Source: CAD feature listing. Evaluate the final solid. Frame: model axes, mm. A direction names the side the tool comes from. Round coordinates to 2 decimals unless told otherwise and drop trailing zeros. Loops run counter-clockwise (first coordinate to the right, second up) from the corner with the lowest first, then second, coordinate; pieces in that order, holes last. Notation, with made-up numbers: (60.5, 23.25) - (118.5, 23.25) arc R37 ccw to (118.5, 60.25) - close; hole circle Ø4 at (6.25, -29.75). An arc over 180 degrees is marked (long way). One line per question, with ' | ' between items. Start each with the question number.
1. Cut plane A-A (x = 0). Return loops of the section in (y, z).
2. Access query for faces 4 (the flat face through (0, 4.636, 41)), 5 (the cylindrical face through (0.255, -6.345, 41.497)), 6 (the cylindrical face through (3.094, -2.372, 15.653)). Directions: +Z, -Z, +X, -X, +Y, -Y. A direction counts if a zero-diameter tool reaches every point of the face in a straight line with its end or side. Return the directions, or none.
3. Ray query, line 1 (Y direction, x = 0, z = 21); line 2 (Z direction, x = -0.25, y = 7.25); line 3 (Z direction, x = 1, y = -1.5). Return the intervals inside material, ascending.
4. Cut plane B-B (y = 0). Return loops of the section in (x, z).
5. Pin query (flat end, axial travel): pin 1 (2.5 mm diameter, centred on x = -0.5, z = 37.5, fed in from +Y); pin 2 (3 mm diameter, centred on y = -1, z = 28, fed in from -X); pin 3 (0.7 mm diameter, centred on y = 5.5, z = 35.5, fed in from +X). Return the tip coordinate at first contact, or that it passes through.
6. Mould query, pull axis Y, two halves, no side actions, for faces 1 (the flat face through (1.714, 5, 41)), 2 (the flat face through (0, 0, 31.75)), 3 (the cylindrical face through (-1.72, -7.75, 12.52)). Classes: pulls with the +Y half, pulls with the -Y half, needs draft (parallel to the pull), parting line crosses it, or undercut.
7. Cut plane D-D (z = 50). Return loops of the section in (x, y).
8. Cut plane C-C (z = 29). Return loops of the section in (x, y).
```python
from build123d import *

# Parameters (mm, degrees)
SKETCH1_R           = 7.9375
BOSS_EXTRUDE1_DEPTH = 57.15
SKETCH2_R           = 3.8989
CUT_EXTRUDE1_DEPTH  = 31.75
SKETCH3_R           = 8.001
CUT_EXTRUDE2_DEPTH  = 31.75


with BuildPart() as part:
    # Sketch1 → Boss-Extrude1 (new body)
    with BuildSketch(Plane.XY):
        Circle(SKETCH1_R)
    extrude(amount=BOSS_EXTRUDE1_DEPTH)

    # Sketch2 → Cut-Extrude1 (cut)
    with BuildSketch(Plane(origin=(0, 0, 0), x_dir=(-1, 0, 0), z_dir=(0, 0, -1))):
        Circle(SKETCH2_R)
    extrude(amount=-CUT_EXTRUDE1_DEPTH, mode=Mode.SUBTRACT)

    # Sketch3 → Cut-Extrude2 (cut)
    with BuildSketch(Plane.XY.offset(57.15)):
        Circle(SKETCH3_R)
        with BuildLine():
            Line((-1.7145, 4.6355), (1.7145, 4.6355))
            Line((1.7145, 4.6355), (1.7145, 6.114163046))
            ThreePointArc((1.7145, 6.114163046), (0, -6.35), (-1.7145, 6.114163046))
            Line((-1.7145, 6.114163046), (-1.7145, 4.6355))
        make_face(mode=Mode.SUBTRACT)
    extrude(amount=-CUT_EXTRUDE2_DEPTH, mode=Mode.SUBTRACT)


solid = part.part
```
Answers follow:
1) outline: (-7.94, 0) - (-3.9, 0) - (-3.9, 31.75) - (3.9, 31.75) - (3.9, 0) - (7.94, 0) - (7.94, 25.4) - (4.64, 25.4) - (4.64, 57.15) - (-6.35, 57.15) - (-6.35, 25.4) - (-7.94, 25.4) - close
2) face 4: +Z, +Y | face 5: +Z | face 6: -Z
3) line 1: y = -7.94 to -3.9, 3.9 to 7.94 | line 2: z = 0 to 25.4 | line 3: z = 31.75 to 57.15
4) outline: (-7.94, 0) - (-3.9, 0) - (-3.9, 31.75) - (3.9, 31.75) - (3.9, 0) - (7.94, 0) - (7.94, 25.4) - (6.35, 25.4) - (6.35, 57.15) - (-6.35, 57.15) - (-6.35, 25.4) - (-7.94, 25.4) - close
5) pin 1: stops at y = 6.11 | pin 2: stops at x = -6.35 | pin 3: stops at x = 3.71
6) face 1: needs draft | face 2: undercut | face 3: parting line crosses it
7) outline: (-1.71, 4.64) - (-1.71, 6.11) arc R6.35 ccw (long way) to (1.71, 6.11) - (1.71, 4.64) - close
8) outline: (-1.71, 4.64) - (-1.71, 6.11) arc R6.35 ccw (long way) to (1.71, 6.11) - (1.71, 4.64) - close; hole circle Ø7.8 at (0, 0)
